from build123d import *

# Parameters (mm, degrees)
SKETCH1_R             = 3
BOSS_EXTRUDE3_DEPTH   = 4
BOSS_EXTRUDE3_2_DEPTH = 4
SKETCH1_9_W           = 34
SKETCH1_9_H           = 20
BOSS_EXTRUDE4_DEPTH   = 2
CUT_EXTRUDE1_DEPTH    = 34
SKETCH3_R             = 3
BOSS_EXTRUDE5_DEPTH   = 3.5


with BuildPart() as part:
    # Sketch1 → Boss-Extrude3 (new body)
    with BuildSketch(Plane.XY):
        with BuildLine():
            ThreePointArc((0.246000737, 6.031372198), (3.088229566, 1.685373233), (8, 0))
            Line((8, 0), (18.5, 0))
            Line((18.5, 0), (18.5, 20))
            Line((18.5, 20), (8, 20))
            ThreePointArc((8, 20), (3.088229566, 18.314626767), (0.246000737, 13.968627802))
            ThreePointArc((0.246000737, 13.968627802), (-1.254, 10), (0.246000737, 6.031372198))
        make_face()
        with Locations((4.746, 10)):
            Circle(SKETCH1_R, mode=Mode.SUBTRACT)
    extrude(amount=-BOSS_EXTRUDE3_DEPTH)



with BuildPart() as body_2:
    # Sketch1 → Boss-Extrude3 2 (new body)
    with BuildSketch(Plane.XY):
        with BuildLine():
            Line((52.5, 20), (52.5, 0))
            Line((52.5, 0), (63, 0))
            ThreePointArc((63, 0), (67.911770434, 1.685373233), (70.753999263, 6.031372198))
            ThreePointArc((70.753999263, 6.031372198), (72.254, 10), (70.753999263, 13.968627802))
            ThreePointArc((70.753999263, 13.968627802), (67.911770434, 18.314626767), (63, 20))
            Line((63, 20), (52.5, 20))
        make_face()
        with Locations((66.254, 10)):
            Circle(SKETCH1_R, mode=Mode.SUBTRACT)
    extrude(amount=-BOSS_EXTRUDE3_2_DEPTH)


with BuildPart() as part_1:
    add(part.part)

    add(body_2.part)  # Boss-Extrude4 merges body 2
    # Sketch1<9> → Boss-Extrude4 (add)
    with BuildSketch(Plane.XY):
        with Locations((35.5, 10)):
            Rectangle(SKETCH1_9_W, SKETCH1_9_H)
    extrude(amount=-BOSS_EXTRUDE4_DEPTH)

    # Sketch2 → Cut-Extrude1 (cut)
    with BuildSketch(Plane(origin=(18.5, 0, 0), x_dir=(0, 0, -1), z_dir=(1, 0, 0))):
        Polygon((2, 20), (0.5, 20), (2, 7.70719), align=None)
    extrude(amount=CUT_EXTRUDE1_DEPTH, mode=Mode.SUBTRACT)

    # Sketch3 → Boss-Extrude5 (add)
    with BuildSketch(Plane(origin=(18.5, 0, 0), x_dir=(0, 0, -1), z_dir=(1, 0, 0))):
        with BuildLine():
            Line((4, 0), (9, 0))
            ThreePointArc((9, 0), (15, 6), (9, 12))
            Line((9, 12), (4, 12))
            Line((4, 12), (4, 0))
        make_face()
        with Locations((9, 6)):
            Circle(SKETCH3_R, mode=Mode.SUBTRACT)
    boss_extrude5 = extrude(amount=-BOSS_EXTRUDE5_DEPTH)

    # Mirror1: Boss-Extrude5 across plane
    add(boss_extrude5.mirror(Plane(origin=(35.5, 0, 0), x_dir=(0, 0, 1), z_dir=(1, 0, 0))))


solid = part_1.part
Work out the finished part from the listing and answer in its coordinate system (mm). A direction names the side the tool comes from. Give positions to 0.01 mm unless a question says otherwise; leave off trailing zeros. Order: outer loops, then holes, each group sorted by start corner. A loop starts at its lowest first (then second) coordinate and runs counter-clockwise, first axis right, second up. Notation, with made-up numbers: (-21.75, 26.5) -> (23.25, 26.5) arc R33 cw to (23.25, 57.5) -> close; hole circle Ø1 at (-30, -2). An arc over 180 degrees is marked (long way). One line per item, written item: value.
Item 1: Find section D-D, the plane y = 10. Give the vertices of the cut face in (x, z), plus the area to 3 significant figures.
Answer sheet:
outline: (-1.25, -4) -> (1.75, -4) -> (1.75, 0) -> (-1.25, 0) -> close; (7.75, -4) -> (15, -4) -> (15, -13.47) -> (18.5, -13.47) -> (18.5, -1.72) -> (52.5, -1.72) -> (52.5, -13.47) -> (56, -13.47) -> (56, -4) -> (63.25, -4) -> (63.25, 0) -> (7.75, 0) -> close; (69.25, -4) -> (72.25, -4) -> (72.25, 0) -> (69.25, 0) -> close
area: 235 mm²
Item 2: Find section B-B, the plane x = 16. Give the vertices of the cut face in (y, z).
Answer sheet:
outline: (0, -9) arc R6 ccw to (12, -9) -> (12, -4) -> (20, -4) -> (20, 0) -> (0, 0) -> close; hole circle Ø6 at (6, -9)
Item 3: Determine the mould class of faces 5 (the cylindrical face through (-1.254, 10.061, -1.972)), 6 (the flat face through (62, 10, -4)), 7 (the flat face through (18.5, 8, -6)), 8 (the cylindrical face through (63.257, 10.132, -1.972)) for opening direction X: released by +X, released by -X, zero draft, split by the parting line, or undercut.
Answer sheet:
face 5: released by -X
face 6: zero draft
face 7: undercut
face 8: undercut
Item 4: A tool of negligible diameter and unlimited length cuts with its end or side. For faces 1 (the flat face through (35, 4, -2)), 2 (the flat face through (35.26, 13.94, -1.24)), 3 (the flat face through (17, 12, -7)), 4 (the flat face through (15, 3, -11)), from which of +Z, -Z, +X, -X, +Y, -Y can it reach the whole face along a straight path? Write none if from no direction.
Answer sheet:
face 1: -Z, +Y, -Y
face 2: -Z, +Y
face 3: -Z, +X, -X, +Y
face 4: -Z, -X, +Y, -Y
Item 5: Find section A-A, the plane z = -3. Give the vertices of the cut face in (x, y), plus the area to 3 significant figures.
Answer sheet:
outline: (0.25, 6.03) arc R8 ccw to (8, 0) -> (18.5, 0) -> (18.5, 20) -> (8, 20) arc R8 ccw to (0.25, 13.97) arc R6 ccw to start; (52.5, 0) -> (63, 0) arc R8 ccw to (70.75, 6.03) arc R6 ccw to (70.75, 13.97) arc R8 ccw to (63, 20) -> (52.5, 20) -> close; hole circle Ø6 at (4.75, 10); hole circle Ø6 at (66.25, 10)
area: 642 mm²
Item 6: Find section C-C, the plane z = -10.5. Give the vertices of the cut face in (x, y), plus the area to 3 significant figures.
Answer sheet:
outline: (15, 0.19) -> (18.5, 0.19) -> (18.5, 3.4) -> (15, 3.4) -> close; (15, 8.6) -> (18.5, 8.6) -> (18.5, 11.81) -> (15, 11.81) -> close; (52.5, 0.19) -> (56, 0.19) -> (56, 3.4) -> (52.5, 3.4) -> close; (52.5, 8.6) -> (56, 8.6) -> (56, 11.81) -> (52.5, 11.81) -> close
area: 45.0 mm²
Item 7: Straight lines are drawn through the part: probe 1 along X at (y, z) = (4.75, -4.75); probe 2 along Y at (x, z) = (55.1, -9); probe 3 along X at (y, z) = (9.5, -1). For each, find the intervals that lie inside material, in ascending order.
Answer sheet:
probe 1: 15 to 18.5, 52.5 to 56
probe 2: 0 to 3, 9 to 12
probe 3: -1.23 to 1.79, 7.7 to 63.3, 69.21 to 72.23
Item 8: Flat-ended cylindrical pins translate along their axes: P1, Ø4.5, axis at y = 14, z = -5.5, coming from the -X side; P2, Ø1, axis at y = 12.5, z = -3, coming from the +X side; P3, Ø4, axis at x = 16, z = -7, coming from the +Y side. Find the tip coordinate at first contact, or state that the pin passes through.
Answer sheet:
P1: x = -0.79
P2: x = 71.91
P3: y = 12
